Study the drawing (mm; zero at the part's minimum x, y, z) and answer. A direction names the side the tool comes from. Round coordinates to 2 decimals unless told otherwise and drop trailing zeros. Write each loop counter-clockwise with the first axis right and the second up, starting at its lowest first coordinate (ties: lowest second). Pieces come first, ordered by that corner, then holes.
(1) Find the intervals of material crossed by probe 1 along X at (y, z) = (336, 139.5); probe 2 along Y at (x, z) = (160, 158); probe 3 along Y at (x, z) = (181.5, 176.5), in increasing order.
(2) A cutting plane is placed at C-C, the plane y = 354.5. Give the vertices of the cut face in (x, z), and give its area (3 significant figures).
(3) A cutting plane is placed at D-D, the plane y = 185. Give the vertices of the cut face in (x, z), and give its area (3 significant figures).
(4) A cutting plane is placed at A-A, the plane x = 160. Give the vertices of the cut face in (y, z), and give its area (3 significant figures).
(5) The mould has two halves that part along X. Classify the marked faces 1, 2, 3 and 4: +X half, -X half, draft (parallel to the pull), parting line (faces both ways), or undercut.
(6) For the marked faces 5, 6 and 7, determine the directions among +Z, -Z, +X, -X, +Y, -Y from which every point of the face is accessible in a straight line to the end or side of a thin tool.
(7) A cutting plane is placed at B-B, the plane z = 160. Give the vertices of the cut face in (x, y).
(8) Each of these flat-tipped pins is pushed along its axis until it touches: pin 1 Ø8 at (x, y) = (187, 87) entering from -Z; pin 2 Ø4 at (y, z) = (177, 121) entering from -X; pin 3 Ø12 at (y, z) = (217.5, 250.5) entering from +X. Where does it stop, or does it pass through?
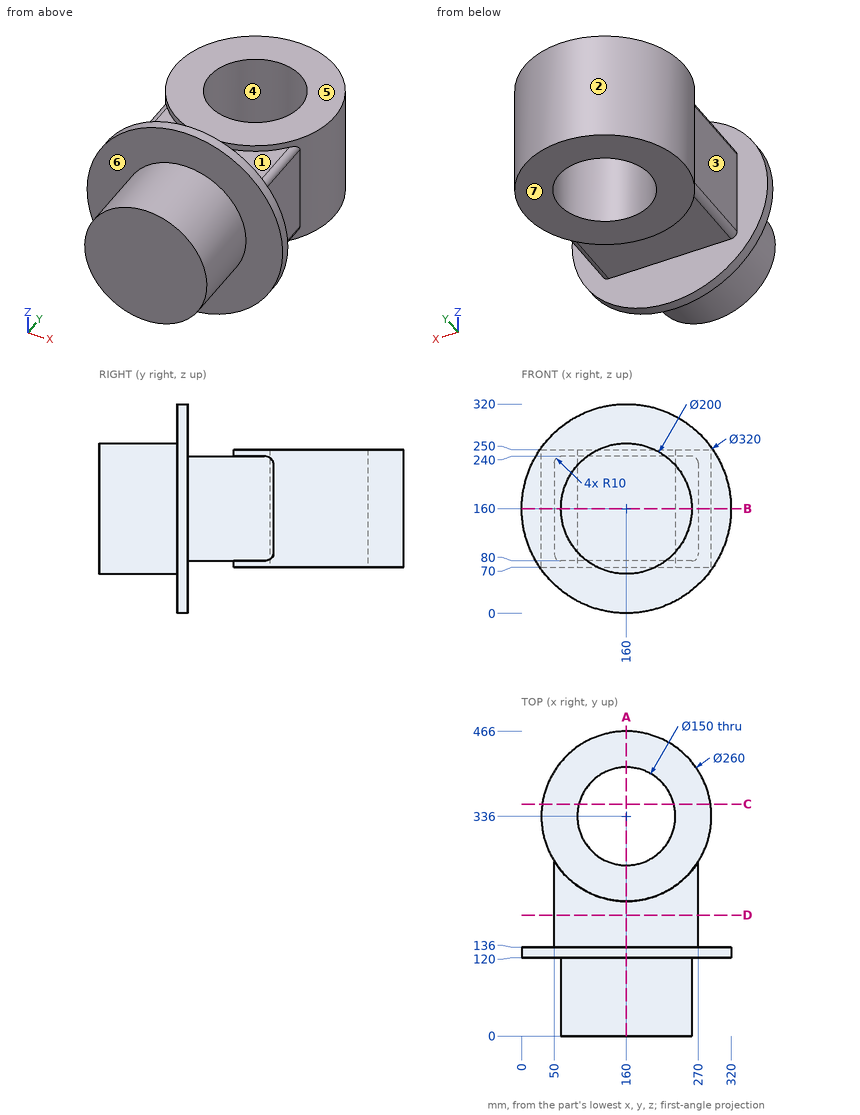
Solutions:
1. probe 1: x = 30 to 85, 235 to 290
1. probe 2: y = 0 to 261, 411 to 466
1. probe 3: y = 0 to 264.15, 407.85 to 464.21
2. outline: (31.32, 70) - (87.32, 70) - (87.32, 250) - (31.32, 250) - close; (232.68, 70) - (288.68, 70) - (288.68, 250) - (232.68, 250) - close
2. area: 20,200 mm2
3. outline: (50, 90) arc R10 ccw to (60, 80) - (260, 80) arc R10 ccw to (270, 90) - (270, 230) arc R10 ccw to (260, 240) - (60, 240) arc R10 ccw to (50, 230) - close
3. area: 35,100 mm2
4. outline: (0, 60) - (120, 60) - (120, 0) - (136, 0) - (136, 80) - (206, 80) - (206, 70) - (261, 70) - (261, 250) - (206, 250) - (206, 240) - (136, 240) - (136, 320) - (120, 320) - (120, 260) - (0, 260) - close; (411, 70) - (466, 70) - (466, 250) - (411, 250) - close
4. area: 60,100 mm2
5. face 1: draft
5. face 2: parting line
5. face 3: -X half
5. face 4: undercut
6. face 5: +Z, +X, -X, +Y
6. face 6: -Y
6. face 7: -Z, +X, -X, +Y
7. outline: (0, 120) - (60, 120) - (60, 0) - (260, 0) - (260, 120) - (320, 120) - (320, 136) - (270, 136) - (270, 266.72) arc R130 ccw (long way) to (50, 266.72) - (50, 136) - (0, 136) - close; hole circle Ø150 at (160, 336)
8. pin 1: stops at z = 62.68
8. pin 2: stops at x = 50
8. pin 3: stops at x = 225.11
